from build123d import *

# Parameters (mm, degrees)
SKETCH1_W           = 45
SKETCH1_H           = 110
BOSS_EXTRUDE1_DEPTH = 3
SKETCH2_R           = 10.95
SKETCH2_R_2         = 15.5
SKETCH2_W           = 24
SKETCH2_H           = 35
CUT_EXTRUDE1_DEPTH  = 4
FILLET1_R           = 4
SKETCH3_W           = 3
SKETCH3_H           = 14
BOSS_EXTRUDE2_DEPTH = 3


with BuildPart() as part:
    # Sketch1 → Boss-Extrude1 (new body)
    with BuildSketch(Plane.XY):
        Rectangle(SKETCH1_W, SKETCH1_H)
    extrude(amount=BOSS_EXTRUDE1_DEPTH)

    # Sketch2 → Cut-Extrude1 (cut, through all)
    with BuildSketch(Plane.XY.offset(3)):
        with Locations((0, -4)):
            Circle(SKETCH2_R)
        with Locations((0, 30.5)):
            Circle(SKETCH2_R_2)
        with Locations((0, -37.5)):
            Rectangle(SKETCH2_W, SKETCH2_H)
        with BuildLine():
            Line((-17.5, 43.5), (-17.5, 48.5))
            ThreePointArc((-17.5, 48.5), (-15.5, 50.5), (-13.5, 48.5))
            Line((-13.5, 48.5), (-13.5, 43.5))
            ThreePointArc((-13.5, 43.5), (-15.5, 41.5), (-17.5, 43.5))
        make_face()
        with BuildLine():
            Line((-13.5, 17.5), (-13.5, 12.5))
            ThreePointArc((-13.5, 12.5), (-15.5, 10.5), (-17.5, 12.5))
            Line((-17.5, 12.5), (-17.5, 17.5))
            ThreePointArc((-17.5, 17.5), (-15.5, 19.5), (-13.5, 17.5))
        make_face()
        with BuildLine():
            Line((17.5, 17.5), (17.5, 12.5))
            ThreePointArc((17.5, 12.5), (15.5, 10.5), (13.5, 12.5))
            Line((13.5, 12.5), (13.5, 17.5))
            ThreePointArc((13.5, 17.5), (15.5, 19.5), (17.5, 17.5))
        make_face()
        with BuildLine():
            Line((13.5, 43.5), (13.5, 48.5))
            ThreePointArc((13.5, 48.5), (15.5, 50.5), (17.5, 48.5))
            Line((17.5, 48.5), (17.5, 43.5))
            ThreePointArc((17.5, 43.5), (15.5, 41.5), (13.5, 43.5))
        make_face()
    extrude(amount=-CUT_EXTRUDE1_DEPTH, mode=Mode.SUBTRACT)

    # Fillet1
    fillet1_edges = [part.edges().sort_by_distance(p)[0] for p in [
        (12, -20, 1.5),
        (-12, -20, 1.5),
    ]]
    fillet(fillet1_edges, radius=FILLET1_R)

    # Sketch3 → Boss-Extrude2 (add)
    with BuildSketch(Plane.XY.offset(3)):
        with Locations((-24, -20)):
            Rectangle(SKETCH3_W, SKETCH3_H)
        with Locations((-24, 8)):
            Rectangle(SKETCH3_W, SKETCH3_H)
        with Locations((-24, -48)):
            Rectangle(SKETCH3_W, SKETCH3_H)
        with Locations((24, -6)):
            Rectangle(SKETCH3_W, SKETCH3_H)
        with Locations((24, -34)):
            Rectangle(SKETCH3_W, SKETCH3_H)
    extrude(amount=-BOSS_EXTRUDE2_DEPTH)


solid = part.part
Can you work these out from the model? Positions are in its coordinate system, mm. A direction names the side the tool comes from. Round coordinates to 2 decimals unless told otherwise and drop trailing zeros. Loops run counter-clockwise (first coordinate to the right, second up) from the corner with the lowest first, then second, coordinate; pieces in that order, holes last. Notation, with made-up numbers: (59.5, 35) - (65.5, 35) arc R12 cw to (65.5, 52) - close; hole circle Ø4 at (-6.75, -30). An arc over 180 degrees is marked (long way). Write item = value, one per line. Start each with the question number.
(1) If we mould it in two halves opening along Y, with no side actions, what happens to faces 5 (the face through (-19, -55, 2)), 6 (the face through (-24, 15, 2)), 7 (the face through (24, -13, 2)), 8 (the face through (-25.5, -48, 2))? For each: released by +Y, released by -Y, zero draft, split by the parting line, or undercut.
(2) If we section it at B-B (y = -4): Please give me the cut outline in (x, z), and give its area (3 significant figures).
(3) If we section it at A-A (x = 0): Please give me the cut outline in (y, z).
(4) For P1, Ø0.9, axis at y = 45, z = 2, coming from the -X side; P2, Ø1.5, axis at y = -19, z = 1.5, coming from the +X side; P3, Ø1.5, axis at x = 23.5, z = 1, coming from the +Y side, each with a flat end and sliding along its axis, tell me the tip position at first contact or that it passes through.
(5) If we section it at D-D (z = 0.5): Give the number of separate pieces and of enclosed holes in the cut face, and give its area (3 significant figures).
(6) For faces 1 (the face through (-15.5, 10.5, 1.5)), 2 (the face through (-22.5, -6, 1)), 3 (the face through (10.859, -21.203, 1.479)), 4 (the face through (24, -27, 2)), which set-ups out of +Z, -Z, +X, -X, +Y, -Y let a thin tool reach every point of the face, with its end or its side?
(7) If I drill on probe 1 along Y at (x, z) = (0, 1); probe 2 along X at (y, z) = (47, 0.85); probe 3 along X at (y, z) = (-38.5, 2.65), over which ranges is the centre line in solid material (lowest first)? Write a range as [from, to].
(8) If we section it at C-C (y = 30.5): Please give me the cut outline in (x, z).
Ans:
q1.face_5 = released by -Y
q1.face_6 = released by +Y
q1.face_7 = undercut
q1.face_8 = zero draft
q2.outline = (-22.5, 0) - (-10.95, 0) - (-10.95, 3) - (-22.5, 3) - close; (10.95, 0) - (25.5, 0) - (25.5, 3) - (10.95, 3) - close
q2.area = 78.3 mm²
q3.outline = (-20, 0) - (-14.95, 0) - (-14.95, 3) - (-20, 3) - close; (6.95, 0) - (15, 0) - (15, 3) - (6.95, 3) - close; (46, 0) - (55, 0) - (55, 3) - (46, 3) - close
q4.P1 = -22.5
q4.P2 = 22.5
q4.P3 = 1
q5.separate_pieces = 1
q5.enclosed_holes = 6
q5.area = 3,070 mm²
q6.face_1 = +Z, -Z
q6.face_2 = +Z, -Z, -X
q6.face_3 = +Z, -Z, -Y
q6.face_4 = +Z, -Z, +X
q7.probe_1 = [-20, -14.95], [6.95, 15], [46, 55]
q7.probe_2 = [-22.5, -17.5], [-13.5, 13.5], [17.5, 22.5]
q7.probe_3 = [-22.5, -12], [12, 25.5]
q8.outline = (-22.5, 0) - (-15.5, 0) - (-15.5, 3) - (-22.5, 3) - close; (15.5, 0) - (22.5, 0) - (22.5, 3) - (15.5, 3) - close
